```python
from build123d import *

# Parameters (mm, degrees)
F0_W     = 50
F0_H     = 50
F0_R     = 2.5
F0_R_2   = 9.55
F1_DEPTH = 15
F3_DEPTH = 25
F4_R     = 10.25
F5_DEPTH = 5


with BuildPart() as f1:
    # F0 (on Top) → F1 (new body)
    with BuildSketch(Plane.XY):
        Rectangle(F0_W, F0_H)
        with Locations((-16.5, -16.5)):
            Circle(F0_R, mode=Mode.SUBTRACT)
        with Locations((16.5, -16.5)):
            Circle(F0_R, mode=Mode.SUBTRACT)
        with Locations((-16.5, 16.5)):
            Circle(F0_R, mode=Mode.SUBTRACT)
        Circle(F0_R_2, mode=Mode.SUBTRACT)
        with Locations((16.5, 16.5)):
            Circle(F0_R, mode=Mode.SUBTRACT)
        Circle(F0_R_2)
    extrude(amount=F1_DEPTH)

    # F2 (on Front) → F3 (cut, symmetric)
    with BuildSketch(Plane.XZ):
        Polygon((25, 15), (-25, 15), (25, 6.183651), align=None)
    extrude(amount=F3_DEPTH, both=True, mode=Mode.SUBTRACT)

    # F4 (on Top) → F5 (cut)
    with BuildSketch(Plane.XY):
        Circle(F4_R)
    extrude(amount=F5_DEPTH, mode=Mode.SUBTRACT)


solid = f1.part
```
Could you check a few things on this model? Use its own coordinates, in mm. A direction names the side the tool comes from. Coordinates: 2 decimals unless noted, no trailing zeros. Write each loop counter-clockwise with the first axis right and the second up, starting at its lowest first coordinate (ties: lowest second). Pieces come first, ordered by that corner, then holes. Notation, with made-up numbers: (-1.75, -5) - (14.25, -5) arc R26 cw to (14.25, 31) - close; hole circle Ø1 at (-39.5, -11). An arc over 180 degrees is marked (long way). Use a Markdown table: item, result.
Q1. Imagine slicing it at D-D (y = -8.5). List the corners of the cut face in (x, z) for me, and give its area (3 significant figures).
Geometry check:
| item | result |
|---|---|
| outline | (-25, 0) - (-5.73, 0) - (-5.73, 5) - (5.73, 5) - (5.73, 0) - (25, 0) - (25, 6.18) - (-25, 15) - close |
| area | 472 mm2 |
Q2. Imagine slicing it at C-C (z = 12). List the corners of the cut face in (x, y) for me.
Geometry check:
| item | result |
|---|---|
| outline | (-25, -25) - (-7.99, -25) - (-7.99, 25) - (-25, 25) - close; hole circle Ø5 at (-16.5, -16.5); hole circle Ø5 at (-16.5, 16.5) |
Q3. Please list where these lines run through material, in increasing order: L1, parallel to Y at x = -16.5, z = 7.5; L2, parallel to Y at x = 18.5, z = 7.
Geometry check:
| item | result |
|---|---|
| L1 | y = -25 to -19, -14 to 14, 19 to 25 |
| L2 | y = -25 to -18, -15 to 15, 18 to 25 |
Q4. Imagine slicing it at A-A (x = -16.5). List the corners of the cut face in (y, z) for me, and give its area (3 significant figures).
Geometry check:
| item | result |
|---|---|
| outline | (-25, 0) - (-19, 0) - (-19, 13.5) - (-25, 13.5) - close; (-14, 0) - (14, 0) - (14, 13.5) - (-14, 13.5) - close; (19, 0) - (25, 0) - (25, 13.5) - (19, 13.5) - close |
| area | 540 mm2 |
Q5. Which directions (+Z, -Z, +X, -X, +Y, -Y) give clear straight access to the entire face, cutting with the end or side of a thin tool? Please do faces 1 (the cylindrical face through (-19, -16.4, 6.9)), 2 (the flat face through (0, 0, 5)).
Geometry check:
| item | result |
|---|---|
| face 1 | +Z, -Z |
| face 2 | -Z |
Q6. I'm going to push flat-ended pins straight in: pin 1 Ø3 at (x, y) = (-8.5, -18.5) entering from +Z; pin 2 Ø6 at (x, y) = (4, 1.5) entering from -Z. Where does each tip first touch, or does it pass through?
Geometry check:
| item | result |
|---|---|
| pin 1 | stops at z = 12.36 |
| pin 2 | stops at z = 5 |
Q7. Imagine slicing it at B-B (y = -16.5). List the corners of the cut face in (x, z) for me, and give its area (3 significant figures).
Geometry check:
| item | result |
|---|---|
| outline | (-25, 0) - (-19, 0) - (-19, 13.94) - (-25, 15) - close; (-14, 0) - (14, 0) - (14, 8.12) - (-14, 13.06) - close; (19, 0) - (25, 0) - (25, 6.18) - (19, 7.24) - close |
| area | 424 mm2 |
Q8. Thinking about a two-plate mould opening in Y: for faces 3 (the flat face through (0, 11, 0)), 4 (the flat face through (-6, -25, 6)), 5 (the cylindrical face through (-2.222, -10.006, 2.465)), which applies, +Y half, -Y half, draft (parallel to the pull), parting line (faces both ways), or undercut?
Geometry check:
| item | result |
|---|---|
| face 3 | draft |
| face 4 | -Y half |
| face 5 | undercut |
